from build123d import *

# Parameters (mm, degrees)
SKETCH1_W                      = 555
SKETCH1_H                      = 100
BASE_FLANGE1_DEPTH             = 1.5
EDGE_FLANGE1_START             = 206.627403552
EDGE_FLANGE1_DEPTH             = 2.426430053
EDGE_FLANGE1_START_2           = -345.946166395
EDGE_FLANGE1_2_DEPTH           = 552.573569947
EDGE_FLANGE1_START_3           = 37.010443104
EDGE_FLANGE1_3_DEPTH           = 97.573569947
EDGE_FLANGE1_4_DEPTH           = 555.946166395
EDGE_FLANGE1_START_4           = 34
EDGE_FLANGE1_5_DEPTH           = 102
EDGE_FLANGE2_START             = 37.010443104
EDGE_FLANGE2_DEPTH             = 97.573569947
EDGE_FLANGE2_START_2           = -345.946166395
EDGE_FLANGE2_2_DEPTH           = 552.573569947
EDGE_FLANGE2_3_DEPTH           = 97.573569947
EDGE_FLANGE2_4_DEPTH           = 552.573569947
EDGE_FLANGE3_STRIP_W           = 7.4732
EDGE_FLANGE3_STRIP_H           = 1.5
EDGE_FLANGE3_STRIP_CUT_DEPTH   = 552.573569946
EDGE_FLANGE3_STRIP_2_W         = 7.4732
EDGE_FLANGE3_STRIP_2_H         = 1.5
EDGE_FLANGE3_STRIP_CUT_2_DEPTH = 97.573569946
EDGE_FLANGE3_DEPTH             = 552.573569946
EDGE_FLANGE3_BEND_DEPTH        = 97.573569946
SKETCH24_R                     = 5
CUT_EXTRUDE1_DEPTH             = 10
LPATTERN1_COUNT                = 2
LPATTERN1_PITCH                = 1005


with BuildPart() as part:
    # Base-Flange1: sheet metal written as solids
    # Sketch1 → Base-Flange1 (new body)
    with BuildSketch(Plane.XY):
        with Locations((-68.446166395, 84.584013051)):
            Rectangle(SKETCH1_W, SKETCH1_H)
    extrude(amount=-BASE_FLANGE1_DEPTH)

    # Edge-Flange1: read off the stored shape, not the designer's step
    # Edge-Flange1 outline → Edge-Flange1 (cut)
    with BuildSketch(Plane.YZ.offset(EDGE_FLANGE1_START)):
        with BuildLine():
            Line((21.941877427, 12.642135624), (35.428928077, -0.844915027))
            ThreePointArc((35.428928077, -0.844915027), (36.154533339, -1.329748962), (37.010443104, -1.5))
            Line((37.010443104, -1.5), (37.010443104, 0))
            ThreePointArc((37.010443104, 0), (36.728558488, 0.056070336), (36.489588249, 0.215745145))
            Line((36.489588249, 0.215745145), (23.002537599, 13.702795796))
            Line((23.002537599, 13.702795796), (21.941877427, 12.642135624))
        make_face()
    extrude(amount=EDGE_FLANGE1_DEPTH, mode=Mode.SUBTRACT)

    # Edge-Flange1 2 outline → Edge-Flange1 2 (add)
    with BuildSketch(Plane.YZ.offset(EDGE_FLANGE1_START_2)):
        with BuildLine():
            Line((21.941877427, 12.642135624), (35.428928077, -0.844915027))
            ThreePointArc((35.428928077, -0.844915027), (36.154533339, -1.329748962), (37.010443104, -1.5))
            Line((37.010443104, -1.5), (37.010443104, 0))
            ThreePointArc((37.010443104, 0), (36.728558488, 0.056070336), (36.489588249, 0.215745145))
            Line((36.489588249, 0.215745145), (23.002537599, 13.702795796))
            Line((23.002537599, 13.702795796), (21.941877427, 12.642135624))
        make_face()
    extrude(amount=EDGE_FLANGE1_2_DEPTH)

    # Edge-Flange1 3 outline → Edge-Flange1 3 (add)
    with BuildSketch(Plane(origin=(0, 0, 0), x_dir=(1, 0, 0), z_dir=(0, 1, 0)).offset(EDGE_FLANGE1_START_3)):
        with BuildLine():
            Line((221.695969229, -12.642135624), (209.053833605, 0))
            Line((209.053833605, 0), (206.627403552, 0))
            ThreePointArc((206.627403552, 0), (206.909288168, -0.056070336), (207.148258407, -0.215745145))
            Line((207.148258407, -0.215745145), (220.635309057, -13.702795796))
            Line((220.635309057, -13.702795796), (221.695969229, -12.642135624))
        make_face()
    extrude(amount=EDGE_FLANGE1_3_DEPTH)

    # Edge-Flange1 4 outline → Edge-Flange1 4 (cut)
    with BuildSketch(Plane.YZ.offset(EDGE_FLANGE1_START_2)):
        with BuildLine():
            ThreePointArc((37.010443104, -1.5), (36.154533339, -1.329748962), (35.428928077, -0.844915027))
            Line((35.428928077, -0.844915027), (34.58401305, 0))
            Line((34.58401305, 0), (34.584013051, -1.5))
            Line((34.584013051, -1.5), (37.010443104, -1.5))
        make_face()
    extrude(amount=EDGE_FLANGE1_4_DEPTH, mode=Mode.SUBTRACT)

    # Edge-Flange1 5 outline → Edge-Flange1 5 (cut)
    with BuildSketch(Plane(origin=(0, 0, 0), x_dir=(1, 0, 0), z_dir=(0, 1, 0)).offset(EDGE_FLANGE1_START_4)):
        with BuildLine():
            ThreePointArc((206.627403552, 1.5), (207.483313316, 1.329748962), (208.208918578, 0.844915027))
            Line((208.208918578, 0.844915027), (209.053833605, 0))
            Line((209.053833605, 0), (209.053833605, 1.5))
            Line((209.053833605, 1.5), (206.627403552, 1.5))
        make_face()
    extrude(amount=EDGE_FLANGE1_5_DEPTH, mode=Mode.SUBTRACT)

    # Edge-Flange2: read off the stored shape, not the designer's step
    # Edge-Flange2 outline → Edge-Flange2 (add)
    with BuildSketch(Plane(origin=(0, 0, 0), x_dir=(1, 0, 0), z_dir=(0, 1, 0)).offset(EDGE_FLANGE2_START)):
        with BuildLine():
            Line((221.695969229, -12.642135624), (239.574648885, -12.642135624))
            Line((239.574648885, -12.642135624), (239.574648885, -11.142135624))
            Line((239.574648885, -11.142135624), (220.501078939, -11.142135624))
            ThreePointArc((220.501078939, -11.142135624), (220.219194323, -11.086065287), (219.980224084, -10.926390479))
            Line((219.980224084, -10.926390479), (221.695969229, -12.642135624))
        make_face()
    extrude(amount=EDGE_FLANGE2_DEPTH)

    # Edge-Flange2 2 outline → Edge-Flange2 2 (add)
    with BuildSketch(Plane.YZ.offset(EDGE_FLANGE2_START_2)):
        with BuildLine():
            Line((23.657622572, 10.926390479), (21.941877427, 12.642135624))
            Line((21.941877427, 12.642135624), (4.06319777, 12.642135624))
            Line((4.06319777, 12.642135624), (4.06319777, 11.142135624))
            Line((4.06319777, 11.142135624), (23.136767717, 11.142135624))
            ThreePointArc((23.136767717, 11.142135624), (23.418652333, 11.086065287), (23.657622572, 10.926390479))
        make_face()
    extrude(amount=EDGE_FLANGE2_2_DEPTH)

    # Edge-Flange2 3 outline → Edge-Flange2 3 (cut)
    with BuildSketch(Plane(origin=(0, 0, 0), x_dir=(1, 0, 0), z_dir=(0, 1, 0)).offset(EDGE_FLANGE2_START)):
        with BuildLine():
            Line((220.635309057, -13.702795796), (221.695969229, -12.642135624))
            Line((221.695969229, -12.642135624), (220.501078939, -12.642135624))
            ThreePointArc((220.501078939, -12.642135624), (219.645169174, -12.471884586), (218.919563912, -11.987050651))
            Line((218.919563912, -11.987050651), (220.635309057, -13.702795796))
        make_face()
    extrude(amount=EDGE_FLANGE2_3_DEPTH, mode=Mode.SUBTRACT)

    # Edge-Flange2 4 outline → Edge-Flange2 4 (cut)
    with BuildSketch(Plane.YZ.offset(EDGE_FLANGE2_START_2)):
        with BuildLine():
            Line((21.941877427, 12.642135624), (23.136767717, 12.642135624))
            ThreePointArc((23.136767717, 12.642135624), (23.992677482, 12.471884586), (24.718282744, 11.987050651))
            Line((24.718282744, 11.987050651), (23.002537599, 13.702795796))
            Line((23.002537599, 13.702795796), (21.941877427, 12.642135624))
        make_face()
    extrude(amount=EDGE_FLANGE2_4_DEPTH, mode=Mode.SUBTRACT)

    # Edge-Flange3: sheet metal written as solids
    # Edge-Flange3 strip (on a plane across the edge) → Edge-Flange3 strip cut (cut)
    with BuildSketch(Plane(origin=(206.627403552, 4.06319777, 11.142135624), x_dir=(0, 1, 0), z_dir=(-1, 0, 0))):
        with Locations((-1.5, -0.75)):
            Rectangle(EDGE_FLANGE3_STRIP_W, EDGE_FLANGE3_STRIP_H)
    extrude(amount=EDGE_FLANGE3_STRIP_CUT_DEPTH, mode=Mode.SUBTRACT)

    # Edge-Flange3 strip 2 (on a plane across the edge) → Edge-Flange3 strip cut 2 (cut)
    with BuildSketch(Plane(origin=(239.574648885, 134.584013051, 11.142135624), x_dir=(-1, 0, 0), z_dir=(0, -1, 0))):
        with Locations((-1.5, -0.75)):
            Rectangle(EDGE_FLANGE3_STRIP_2_W, EDGE_FLANGE3_STRIP_2_H)
    extrude(amount=EDGE_FLANGE3_STRIP_CUT_2_DEPTH, mode=Mode.SUBTRACT)

    # Edge-Flange3 section (on a plane across the edge) → Edge-Flange3 (add)
    with BuildSketch(Plane(origin=(206.627403552, 4.06319777, 11.142135624), x_dir=(0, 1, 0), z_dir=(-1, 0, 0))):
        with BuildLine():
            Line((0, 0.7366), (0, 13.5))
            Line((0, 13.5), (1.5, 13.5))
            Line((1.5, 13.5), (1.5, 0.7366))
            ThreePointArc((1.5, 0.7366), (1.715745145, 0.215745145), (2.2366, 0))
            Line((2.2366, 0), (2.2366, -1.5))
            ThreePointArc((2.2366, -1.5), (0.655084973, -0.844915027), (0, 0.7366))
        make_face()
    extrude(amount=EDGE_FLANGE3_DEPTH)

    # Edge-Flange3 section 2 (on a plane across the edge) → Edge-Flange3 bend (add)
    with BuildSketch(Plane(origin=(239.574648885, 134.584013051, 11.142135624), x_dir=(-1, 0, 0), z_dir=(0, -1, 0))):
        with BuildLine():
            Line((0, 0.7366), (0, 13.5))
            Line((0, 13.5), (1.5, 13.5))
            Line((1.5, 13.5), (1.5, 0.7366))
            ThreePointArc((1.5, 0.7366), (1.715745145, 0.215745145), (2.2366, 0))
            Line((2.2366, 0), (2.2366, -1.5))
            ThreePointArc((2.2366, -1.5), (0.655084973, -0.844915027), (0, 0.7366))
        make_face()
    extrude(amount=EDGE_FLANGE3_BEND_DEPTH)

    # Mirror1: part across plane


with BuildPart() as part_1:
    add(part.part)
    add(part.part.mirror(Plane(origin=(-345.946166395, 134.584013051, -1.5), x_dir=(0, 0, 1), z_dir=(-1, 0, 0))))

    # Mirror2: part across plane


with BuildPart() as part_2:
    add(part_1.part)
    add(part_1.part.mirror(Plane(origin=(-345.946166395, 134.584013051, -1.5), x_dir=(0, 0, 1), z_dir=(0, 1, 0))))

    # Sketch24 → Cut-Extrude1 (cut)
    with BuildSketch(Plane.XY):
        with Locations((-851.466981675, 119.06319777)):
            Circle(SKETCH24_R)
    cut_extrude1 = extrude(amount=-CUT_EXTRUDE1_DEPTH, mode=Mode.SUBTRACT)

    # LPattern1: Cut-Extrude1 ×2
    with Locations(*[(i * LPATTERN1_PITCH, 0, 0) for i in range(1, LPATTERN1_COUNT)]):
        add(cut_extrude1, mode=Mode.SUBTRACT)


solid = part_2.part
For this review, take the finished solid that the model builds, in its own axes (mm). A direction names the side the tool comes from. Round coordinates to 2 decimals unless told otherwise and drop trailing zeros. Order: outer loops, then holes, each group sorted by start corner. A loop starts at its lowest first (then second) coordinate and runs counter-clockwise, first axis right, second up. Notation, with made-up numbers: M 31.5,-35 L 76.5,-35 A29 ccw 76.5,1 Z; hole C 38.5,43.25 d7. An arc over 180 degrees is marked long. Use a Markdown table: item, result. Add a question column.
Item 1: Insertion check: pin 1 (11.5 mm diameter, centred on x = -851.47, y = 119.06, fed in from +Z); pin 2 (8.5 mm diameter, centred on x = -124.5, y = 253, fed in from -Z); pin 3 (1.5 mm diameter, centred on x = 26, y = 111, fed in from -Z). Each pin has a flat end and moves straight along its axis. Give the tip position at first contact, or say it passes through.
Item 2: Add section C-C, the plane z = 6.75. State how many separate pieces and enclosed holes the cut face has, then the cut area to 3 significant figures.
Item 3: Add section B-B, the plane x = -663. Give the boundary of the cut face in (y, z), then the cut area to 3 significant figures.
Item 4: Add section A-A, the plane y = 211. Give the boundary of the cut face in (x, z), then the cut area to 3 significant figures.
Item 5: To check wall thickness, follow line 1 along X through (y, z) = (97, 0.25); line 2 along X through (y, z) = (141.5, 7.5); line 3 along Y through (x, z) = (-227.5, -0.25). State the ranges of each line that lie inside material, in increasing order.
Item 6: Tool access review of faces 1 (the flat face through (-338, 133, -1.5)), 2 (the flat face through (-338, 133, 0)): name each direction out of +Z, -Z, +X, -X, +Y, -Y from which nothing blocks a thin tool from reaching the whole face with its end or side.
Geometry results:
| question | item | result |
|---|---|---|
| 1 | pin 1 | stops at z = 0 |
| 1 | pin 2 | stops at z = 11.14 |
| 1 | pin 3 | stops at z = -1.5 |
| 2 | separate pieces | 8 |
| 2 | enclosed holes | 0 |
| 2 | area | 9,420 mm² |
| 3 | outline | M 4.06,-2.36 L 5.56,-2.36 L 5.56,10.41 A0.74 cw 6.3,11.14 L 23.14,11.14 A0.74 cw 23.66,10.93 L 35.43,-0.84 A2.24 ccw 37.01,-1.5 L 232.16,-1.5 A2.24 ccw 233.74,-0.84 L 245.51,10.93 A0.74 cw 246.03,11.14 L 262.87,11.14 A0.74 cw 263.6,10.41 L 263.6,-2.36 L 265.1,-2.36 L 265.1,10.41 A2.24 ccw 262.87,12.64 L 246.03,12.64 A2.24 ccw 244.45,11.99 L 232.68,0.22 A0.74 cw 232.16,0 L 37.01,0 A0.74 cw 36.49,0.22 L 24.72,11.99 A2.24 ccw 23.14,12.64 L 6.3,12.64 A2.24 ccw 4.06,10.41 Z |
| 3 | area | 445 mm² |
| 4 | outline | M -931.47,-2.36 L -929.97,-2.36 L -929.97,10.41 A0.74 cw -929.23,11.14 L -912.39,11.14 A0.74 cw -911.87,10.93 L -900.1,-0.84 A2.24 ccw -898.52,-1.5 L 206.63,-1.5 A2.24 ccw 208.21,-0.84 L 219.98,10.93 A0.74 cw 220.5,11.14 L 237.34,11.14 A0.74 cw 238.07,10.41 L 238.07,-2.36 L 239.57,-2.36 L 239.57,10.41 A2.24 ccw 237.34,12.64 L 220.5,12.64 A2.24 ccw 218.92,11.99 L 207.15,0.22 A0.74 cw 206.63,0 L -898.52,0 A0.74 cw -899.04,0.22 L -910.81,11.99 A2.24 ccw -912.39,12.64 L -929.23,12.64 A2.24 ccw -931.47,10.41 Z |
| 4 | area | 1,810 mm² |
| 5 | line 1 | x = -931.47 to -929.97, -901.2 to -899.07, 207.18 to 209.3, 238.07 to 239.57 |
| 5 | line 2 | x = -931.47 to -929.97, -908.45 to -906.32, 214.43 to 216.55, 238.07 to 239.57 |
| 5 | line 3 | y = 4.06 to 5.56, 34.83 to 234.33, 263.6 to 265.1 |
| 6 | face 1 | -Z |
| 6 | face 2 | +Z |
